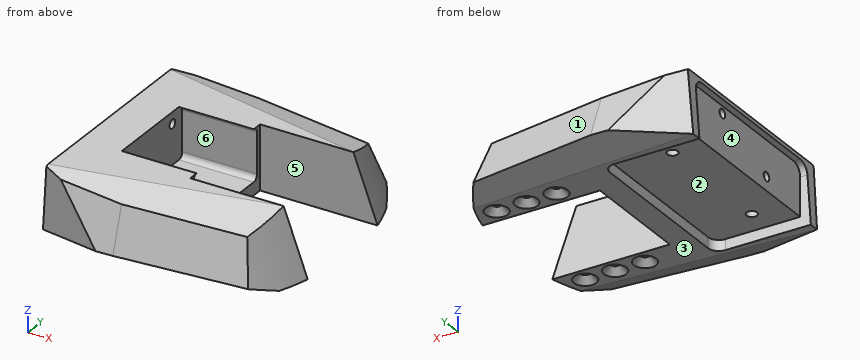
from build123d import *

# Parameters (mm, degrees)
BOSS_EXTRUDE1_DEPTH             = 30
SKETCH3_W                       = 30
SKETCH3_H                       = 52.601373674
CUT_EXTRUDE1_DEPTH              = 20
DRAFT1_ANGLE                    = 20
CUT_EXTRUDE2_DEPTH              = 5
CUT_EXTRUDE3_DEPTH              = 5
M6X1_0_TAPPED_HOLE1_D           = 5
M6X1_0_TAPPED_HOLE1_DEPTH       = 10
M6X1_0_TAPPED_HOLE1_TIP         = 1.502151548
CUT_REVOLVE1_ANGLE              = 20
CUT_REVOLVE2_ANGLE              = 20
CUT_REVOLVE3_ANGLE              = 20
CUT_REVOLVE4_ANGLE              = 20
CUT_EXTRUDE4_DEPTH              = 35
M5X0_8_TAPPED_HOLE1_D           = 4.2
SKETCH19_W                      = 47.516094142
SKETCH19_H                      = 117.781056104
CUT_REVOLVE5_ANGLE              = 4
M5X0_8_TAPPED_HOLE2_D           = 4.2
M5X0_8_TAPPED_HOLE2_DEPTH       = 10
M5X0_8_TAPPED_HOLE2_CSINK_D     = 10.5
M5X0_8_TAPPED_HOLE2_CSINK_ANGLE = 90
M5X0_8_TAPPED_HOLE2_TIP         = 1.2618073


with BuildPart() as part:
    # Sketch2 → Boss-Extrude1 (new body)
    with BuildSketch(Plane.XY):
        with BuildLine():
            Line((-41.221662469, 50), (-50, 46.630311934))
            Line((-50, 46.630311934), (-50, -46.630311934))
            Line((-50, -46.630311934), (-41.221662469, -50))
            Line((-41.221662469, -50), (-10.163742616, -50))
            Line((-10.163742616, -50), (43.420662363, -43.420662363))
            ThreePointArc((43.420662363, -43.420662363), (47.113322701, -35.015547326), (50, -26.300686837))
            Line((50, -26.300686837), (26.300686837, -26.300686837))
            Line((26.300686837, -26.300686837), (26.300686837, 26.300686837))
            Line((26.300686837, 26.300686837), (50, 26.300686837))
            ThreePointArc((50, 26.300686837), (47.113322701, 35.015547326), (43.420662363, 43.420662363))
            Line((43.420662363, 43.420662363), (-10.163742616, 50))
            Line((-10.163742616, 50), (-41.221662469, 50))
        make_face()
    extrude(amount=BOSS_EXTRUDE1_DEPTH)

    # Sketch3 → Cut-Extrude1 (cut)
    with BuildSketch(Plane(origin=(26.300686837, 0, 0), x_dir=(0, 0, -1), z_dir=(1, 0, 0))):
        with Locations((-15, 0)):
            Rectangle(SKETCH3_W, SKETCH3_H)
    extrude(amount=-CUT_EXTRUDE1_DEPTH, mode=Mode.SUBTRACT)

    # Draft1
    draft1_faces = [part.faces().sort_by_distance(p)[0] for p in [
        (-25.692702542, 50, 15),
        (16.628459874, 46.710331182, 15),
        (47.113322701, 35.015547326, 15),
        (47.113322701, -35.015547326, 15),
        (-25.692702542, -50, 15),
        (16.628459874, -46.710331182, 15),
    ]]
    draft(draft1_faces, Plane.XY.offset(30), DRAFT1_ANGLE)

    # Sketch5 → Cut-Extrude2 (cut)
    with BuildSketch(Plane.ZY.offset(50)):
        with BuildLine():
            Line((0, 42), (23, 42))
            ThreePointArc((23, 42), (26.535533906, 40.535533906), (28, 37))
            Line((28, 37), (28, -37))
            ThreePointArc((28, -37), (26.535533906, -40.535533906), (23, -42))
            Line((23, -42), (0, -42))
            Line((0, -42), (0, 42))
        make_face()
    extrude(amount=-CUT_EXTRUDE2_DEPTH, mode=Mode.SUBTRACT)

    # Sketch6 → Cut-Extrude3 (cut)
    with BuildSketch(Plane(origin=(0, 0, 0), x_dir=(-1, 0, 0), z_dir=(0, 0, -1))):
        with BuildLine():
            Line((45, 42), (10, 42))
            ThreePointArc((10, 42), (6.464466094, 40.535533906), (5, 37))
            Line((5, 37), (5, -37))
            ThreePointArc((5, -37), (6.464466094, -40.535533906), (10, -42))
            Line((10, -42), (45, -42))
            Line((45, -42), (45, 42))
        make_face()
    extrude(amount=-CUT_EXTRUDE3_DEPTH, mode=Mode.SUBTRACT)

    # M6x1.0 Tapped Hole1
    with Locations(Plane(origin=(0, 0, 5), x_dir=(-1, 0, 0), z_dir=(0, 0, -1))):
        with Locations((29.9, 29.895651858), (29.9, -29.895651858)):
            Hole(M6X1_0_TAPPED_HOLE1_D / 2, depth=M6X1_0_TAPPED_HOLE1_DEPTH)
            with Locations((0, 0, -(M6X1_0_TAPPED_HOLE1_DEPTH + M6X1_0_TAPPED_HOLE1_TIP / 2))):  # 118° drill point
                Cone(0, M6X1_0_TAPPED_HOLE1_D / 2, M6X1_0_TAPPED_HOLE1_TIP, mode=Mode.SUBTRACT)

    # Sketch9 → Cut-Revolve1 (revolve, cut)
    with BuildSketch(Plane(origin=(0, 0, 0), x_dir=(-1, 0, 0), z_dir=(0, 0, -1))):
        with BuildLine():
            Line((50, 46.630311934), (-56.76790933, 40.30398391))
            ThreePointArc((-56.76790933, 40.30398391), (-54.419330105, 48.540812289), (-51.472316128, 56.582968389))
            Line((-51.472316128, 56.582968389), (18.167108014, 64.912852718))
            Line((18.167108014, 64.912852718), (50, 46.630311934))
        make_face()
    revolve(axis=Axis((-50, 46.630311934, 0), (0.9982491449473906, -0.0591493416007627, 0)), revolution_arc=CUT_REVOLVE1_ANGLE, mode=Mode.SUBTRACT)

    # Sketch11 → Cut-Revolve2 (revolve, cut)
    with BuildSketch(Plane(origin=(0, 0, 0), x_dir=(-1, 0, 0), z_dir=(0, 0, -1))):
        with BuildLine():
            Line((50, -46.630311934), (-56.76790933, -40.30398391))
            ThreePointArc((-56.76790933, -40.30398391), (-55.407295575, -48.597993011), (-53.453959647, -56.772730652))
            Line((-53.453959647, -56.772730652), (21.223580117, -65.428953237))
            Line((21.223580117, -65.428953237), (50, -46.630311934))
        make_face()
    revolve(axis=Axis((-50, -46.630311934, 0), (-0.9982491449473906, -0.05914934160076277, 0)), revolution_arc=CUT_REVOLVE2_ANGLE, mode=Mode.SUBTRACT)

    # Sketch13 → Cut-Revolve3 (revolve, cut)
    with BuildSketch(Plane.XY.offset(30)):
        Polygon((-50, 46.630311934), (50, 26.300686837), (49.446951964, 52.159989852), (-50, 58.994858097), align=None)
    revolve(axis=Axis((-50, 46.630311934, 30), (-0.9799545689980745, 0.1992210899975155, 0)), revolution_arc=CUT_REVOLVE3_ANGLE, mode=Mode.SUBTRACT)

    # Sketch14 → Cut-Revolve4 (revolve, cut)
    with BuildSketch(Plane.XY.offset(30)):
        Polygon((50, -26.300686837), (49.446951964, -52.159989852), (-50, -58.995311934), (-50, -46.630311934), align=None)
    revolve(axis=Axis((50, -26.300686837, 30), (0.9799545689980745, 0.1992210899975155, 0)), revolution_arc=CUT_REVOLVE4_ANGLE, mode=Mode.SUBTRACT)

    # Sketch15 → Cut-Extrude4 (cut)
    with BuildSketch(Plane(origin=(6.300686837, 0, 0), x_dir=(0, 0, -1), z_dir=(1, 0, 0))):
        with BuildLine():
            Line((-30, 0), (-30, -21.5))
            ThreePointArc((-30, -21.5), (-29.267766953, -23.267766953), (-27.5, -24))
            Line((-27.5, -24), (-8.5, -24))
            ThreePointArc((-8.5, -24), (-6.732233047, -23.267766953), (-6, -21.5))
            Line((-6, -21.5), (-6, 21.5))
            ThreePointArc((-6, 21.5), (-6.732233047, 23.267766953), (-8.5, 24))
            Line((-8.5, 24), (-27.5, 24))
            ThreePointArc((-27.5, 24), (-29.267766953, 23.267766953), (-30, 21.5))
            Line((-30, 21.5), (-30, 0))
        make_face()
    extrude(amount=-CUT_EXTRUDE4_DEPTH, mode=Mode.SUBTRACT)

    # M5x0.8 Tapped Hole1 (through all)
    with Locations(Plane(origin=(-28.699313163, 0, 0), x_dir=(0, 0, -1), z_dir=(1, 0, 0))):
        with Locations((-11.497988924, -16.605361405), (-24.602011076, 16.605361405)):
            Hole(M5X0_8_TAPPED_HOLE1_D / 2)

    # Sketch19 → Cut-Revolve5 (revolve, cut)
    with BuildSketch(Plane.ZY.offset(50)):
        with Locations((23.758047071, 0)):
            Rectangle(SKETCH19_W, SKETCH19_H)
    revolve(axis=Axis((-50, 58.890528052, 0), (0, 1, 0)), revolution_arc=CUT_REVOLVE5_ANGLE, mode=Mode.SUBTRACT)

    # M5x0.8 Tapped Hole2
    with Locations(Plane(origin=(0, 0, 0), x_dir=(-1, 0, 0), z_dir=(0, 0, -1))):
        with Locations((-50.268656574, 33.379143774), (-50.268656574, -33.379143774), (-36.268656574, -33.379143774), (-22.268656574, -33.379143774), (-36.268656574, 33.379143774), (-22.268656574, 33.379143774)):
            CounterSinkHole(M5X0_8_TAPPED_HOLE2_D / 2, M5X0_8_TAPPED_HOLE2_CSINK_D / 2, depth=M5X0_8_TAPPED_HOLE2_DEPTH, counter_sink_angle=M5X0_8_TAPPED_HOLE2_CSINK_ANGLE)
            with Locations((0, 0, -(M5X0_8_TAPPED_HOLE2_DEPTH + M5X0_8_TAPPED_HOLE2_TIP / 2))):  # 118° drill point
                Cone(0, M5X0_8_TAPPED_HOLE2_D / 2, M5X0_8_TAPPED_HOLE2_TIP, mode=Mode.SUBTRACT)


solid = part.part
The listing builds one solid part. Answer for the finished solid, in the listing's coordinates (mm). Face numbers are marked on the shaded views. A direction names the side the tool comes from. Give positions to 0.01 mm unless a question says otherwise; leave off trailing zeros. Order: outer loops, then holes, each group sorted by start corner. A loop starts at its lowest first (then second) coordinate and runs counter-clockwise, first axis right, second up. Notation, with made-up numbers: (-1, -8.5) - (33, -8.5) arc R19 cw to (33, 10.5) - close; hole circle Ø8 at (29, 31). An arc over 180 degrees is marked (long way). One line per item, written item: value. Start each with the question number.
1) Given pin 1 Ø2 at (x, y) = (-26.5, 11) entering from -Z; pin 2 Ø5.5 at (y, z) = (5, 1.5) entering from -X; pin 3 Ø15 at (x, z) = (-13.5, 16) entering from +Y, each flat-ended and moving along its own axis, determine where each tip first touches the part or whether it passes through.
2) A cutting plane is placed at C-C on x = -20. Give the vertices of the cut face in (y, z), then the cut area to 3 significant figures.
3) The mould has two halves that part along Y. Classify the marked faces 1, 2 and 3: released by +Y, released by -Y, zero draft, split by the parting line, or undercut.
4) A cutting plane is placed at D-D on x = -1. Give the vertices of the cut face in (y, z), then the cut area to 3 significant figures.
5) A cutting plane is placed at A-A on x = -36.5. Give the vertices of the cut face in (y, z).
6) Find the intervals of material crossed by L1, parallel to Z at x = -37, y = 25; L2, parallel to Y at x = 40, z = 11.5; L3, parallel to Z at x = 16.5, y = -40.5, in increasing order.
7) A tool of negligible diameter and unlimited length cuts with its end or side. For the marked faces 4, 5 and 6, from which of +Z, -Z, +X, -X, +Y, -Y can it reach the whole face along a straight path? Write none if from no direction.
8) A cutting plane is placed at B-B on z = 18. Give the vertices of the cut face in (x, y).
Answer sheet:
1. pin 1: stops at z = 5
1. pin 2: stops at x = -5
1. pin 3: stops at y = 57.83
2. outline: (-58.15, 4.83) - (-44.85, 0) - (-42, 0) - (-42, 5) - (42, 5) - (42, 0) - (44.85, 0) - (58.15, 4.83) - (58.15, 7.62) - (51.41, 26.12) - (40.53, 30) - (21.5, 30) arc R2.5 cw to (24, 27.5) - (24, 8.5) arc R2.5 cw to (21.5, 6) - (-21.5, 6) arc R2.5 cw to (-24, 8.5) - (-24, 27.5) arc R2.5 cw to (-21.5, 30) - (-40.53, 30) - (-51.41, 26.12) - (-58.15, 7.62) - close
2. area: 1,640 mm2
3. face 1: released by +Y
3. face 2: undercut
3. face 3: zero draft
4. outline: (-57.98, 5.18) - (-43.73, 0) - (43.73, 0) - (57.98, 5.18) - (50.71, 24.99) - (36.67, 30) - (21.5, 30) arc R2.5 cw to (24, 27.5) - (24, 8.5) arc R2.5 cw to (21.5, 6) - (-21.5, 6) arc R2.5 cw to (-24, 8.5) - (-24, 27.5) arc R2.5 cw to (-21.5, 30) - (-36.67, 30) - (-50.71, 24.99) - close
4. area: 1,970 mm2
5. outline: (-51.81, 2.17) - (-45.83, 0) - (-42, 0) - (-42, 5) - (42, 5) - (42, 0) - (45.83, 0) - (51.81, 2.17) - (51.81, 25.02) - (50.91, 27.49) - (43.89, 30) - (-43.89, 30) - (-50.91, 27.49) - (-51.81, 25.02) - close; hole circle Ø4.2 at (-16.61, 11.5); hole circle Ø4.2 at (16.61, 24.6)
6. L1: z = 5 to 30
6. L2: y = -50.62 to -26.3, 26.3 to 50.62
6. L3: z = 0 to 27.36
7. face 4: -Z, -X
7. face 5: +Z, -Z, +X
7. face 6: +X
8. outline: (-48.74, -47.11) - (-29.84, -54.37) - (-9.9, -54.37) - (46.25, -47.47) arc R101.98 ccw to (54.53, -26.3) - (6.3, -26.3) - (6.3, -24) - (-28.7, -24) - (-28.7, 24) - (6.3, 24) - (6.3, 26.3) - (54.53, 26.3) arc R101.98 ccw to (46.25, 47.47) - (-9.9, 54.37) - (-29.84, 54.37) - (-48.74, 47.11) - (-48.74, 42) - (-45, 42) - (-45, -42) - (-48.74, -42) - close
